Verification items for the finished model (mm, model axes). A direction names the side the tool comes from. Give positions to 0.01 mm unless a question says otherwise; leave off trailing zeros. Order: outer loops, then holes, each group sorted by start corner. A loop starts at its lowest first (then second) coordinate and runs counter-clockwise, first axis right, second up.
from build123d import *

# Parameters (mm, degrees)
BOSS_EXTRUDE1_DEPTH = 70
SKETCH3_R           = 19.5
BOSS_EXTRUDE2_DEPTH = 23
CUT_EXTRUDE1_DEPTH  = 23
CUT_EXTRUDE2_DEPTH  = 12
SKETCH4_W           = 22
SKETCH4_H           = 92.60205789
CUT_EXTRUDE3_DEPTH  = 6
SKETCH5_W           = 22
SKETCH5_H           = 56
CUT_EXTRUDE4_DEPTH  = 6


with BuildPart() as part:
    # Sketch1 → Boss-Extrude1 (new body)
    with BuildSketch(Plane(origin=(0, 0, 0), x_dir=(0, 0, -1), z_dir=(1, 0, 0))):
        Polygon((0, 0), (-149.274923862, 0), (-212.764789027, 75.664274903), (-191.31554462, 93.662327975), (-206.099659643, 111.281350166), (-245.167926242, 78.499182072), (-160, -23), (0, -23), align=None)
    extrude(amount=-BOSS_EXTRUDE1_DEPTH)

    # Sketch3 → Boss-Extrude2 (add)
    with BuildSketch(Plane(origin=(0, 166.78684827, 139.950782869), x_dir=(1, 0, 0), z_dir=(0, 0.766044443, 0.64278761))):
        with Locations((-35, -86.351225922)):
            Circle(SKETCH3_R)
        with BuildLine():
            ThreePointArc((-70, -86.351225922), (-35, -51.351225922), (0, -86.351225922))
            Line((0, -86.351225922), (-70, -86.351225922))
        make_face()
        with BuildLine():
            Line((-44.5, -86.351225922), (-54.5, -86.351225922))
            ThreePointArc((-54.5, -86.351225922), (-35, -105.851225922), (-15.5, -86.351225922))
            Line((-15.5, -86.351225922), (-25.5, -86.351225922))
            ThreePointArc((-25.5, -86.351225922), (-35, -95.851225922), (-44.5, -86.351225922))
        make_face()
        with BuildLine():
            ThreePointArc((-15.5, -86.351225922), (-35, -66.851225922), (-54.5, -86.351225922))
            Line((-54.5, -86.351225922), (-44.5, -86.351225922))
            ThreePointArc((-44.5, -86.351225922), (-35, -76.851225922), (-25.5, -86.351225922))
            Line((-25.5, -86.351225922), (-15.5, -86.351225922))
        make_face()
    extrude(amount=-BOSS_EXTRUDE2_DEPTH)

    # Sketch3_3 → Cut-Extrude1 (cut)
    with BuildSketch(Plane(origin=(0, 166.78684827, 139.950782869), x_dir=(1, 0, 0), z_dir=(0, 0.766044443, 0.64278761))):
        with BuildLine():
            Line((-25.5, -86.351225922), (-44.5, -86.351225922))
            ThreePointArc((-44.5, -86.351225922), (-35, -95.851225922), (-25.5, -86.351225922))
        make_face()
        with BuildLine():
            ThreePointArc((-25.5, -86.351225922), (-35, -76.851225922), (-44.5, -86.351225922))
            Line((-44.5, -86.351225922), (-25.5, -86.351225922))
        make_face()
    extrude(amount=-CUT_EXTRUDE1_DEPTH, mode=Mode.SUBTRACT)

    # Sketch3_4 → Cut-Extrude2 (cut)
    with BuildSketch(Plane(origin=(0, 166.78684827, 139.950782869), x_dir=(1, 0, 0), z_dir=(0, 0.766044443, 0.64278761))):
        with BuildLine():
            Line((-44.5, -86.351225922), (-54.5, -86.351225922))
            ThreePointArc((-54.5, -86.351225922), (-35, -105.851225922), (-15.5, -86.351225922))
            Line((-15.5, -86.351225922), (-25.5, -86.351225922))
            ThreePointArc((-25.5, -86.351225922), (-35, -95.851225922), (-44.5, -86.351225922))
        make_face()
        with BuildLine():
            ThreePointArc((-15.5, -86.351225922), (-35, -66.851225922), (-54.5, -86.351225922))
            Line((-54.5, -86.351225922), (-44.5, -86.351225922))
            ThreePointArc((-44.5, -86.351225922), (-35, -76.851225922), (-25.5, -86.351225922))
            Line((-25.5, -86.351225922), (-15.5, -86.351225922))
        make_face()
    extrude(amount=-CUT_EXTRUDE2_DEPTH, mode=Mode.SUBTRACT)

    # Sketch4 → Cut-Extrude3 (cut)
    with BuildSketch(Plane(origin=(0, 166.78684827, 139.950782869), x_dir=(1, 0, 0), z_dir=(0, 0.766044443, 0.64278761))):
        with Locations((-35, -91.050196977)):
            Rectangle(SKETCH4_W, SKETCH4_H)
    extrude(amount=-CUT_EXTRUDE3_DEPTH, mode=Mode.SUBTRACT)

    # Sketch5 → Cut-Extrude4 (cut)
    with BuildSketch(Plane(origin=(0, -88.287666198, 105.217143373), x_dir=(1, 0, 0), z_dir=(0, -0.64278761, 0.766044443))):
        with Locations((-35, 183.724767497)):
            Rectangle(SKETCH5_W, SKETCH5_H)
    extrude(amount=-CUT_EXTRUDE4_DEPTH, mode=Mode.SUBTRACT)


solid = part.part
(1) Section check A-A, the plane x = -28. Enter the section's corners in (y, z).
Solved:
outline: (-23, 0) - (0, 0) - (0, 149.27) - (75.66, 212.76) - (89.53, 196.24) - (97.96, 203.31) - (90.39, 212.33) - (94.99, 216.19) - (77.76, 236.71) - (34.86, 200.72) - (31, 205.32) - (-23, 160) - close; (97.79, 186.4) - (115.71, 165.05) - (128.73, 175.97) - (118.38, 188.3) - (113.79, 184.44) - (106.22, 193.47) - close
(2) Section check C-C, the plane x = -41.5. Enter the section's corners in (y, z), then the cut area to 3 significant figures.
Solved:
outline: (-23, 0) - (0, 0) - (0, 149.27) - (75.66, 212.76) - (89.21, 196.62) - (97.64, 203.69) - (90.27, 212.47) - (94.87, 216.33) - (77.76, 236.71) - (34.86, 200.72) - (31, 205.32) - (-23, 160) - close; (98.12, 186.01) - (115.77, 164.97) - (128.79, 175.9) - (118.5, 188.16) - (113.91, 184.3) - (106.54, 193.08) - close
area: 6,690 mm2
(3) Section check D-D, the plane z = 95. Enter the section's corners in (x, y).
Solved:
outline: (-70, -23) - (0, -23) - (0, 0) - (-70, 0) - close
(4) Scan lines: line 1 (Y direction, x = -57.5, z = 27.5); line 2 (Z direction, x = -59, y = 91.5); line 3 (Z direction, x = -17, y = -5). Record each from-to range of solid material in increasing order.
Solved:
line 1: y = -23 to 0
line 2: z = 193.89 to 229.67
line 3: z = 0 to 175.1
(5) Set-up check for faces 4 (the flat face through (-35.154, 123.194, 182.569)), 5 (the flat face through (-46, 65.6, 226.8)), 6 (the flat face through (-34.51, 37.302, 180.575)), 7 (the flat face through (-43.94, 99.479, 201.497)), 8 (the flat face through (-35, 0, 74)): record each of +Z, -Z, +X, -X, +Y, -Y from which the full face is reachable in a straight line by a thin tool's end or side.
Solved:
face 4: +Z, +Y
face 5: +Z
face 6: -Z, +X, -X
face 7: none
face 8: -Z, +X, -X, +Y
(6) Release check for a two-part mould opening along X. For faces 1 (the cylindrical face through (-35.77, 125.09, 172.01)), 2 (the cylindrical face through (-37.06, 91.97, 202)), 3 (the flat face through (-35, -12, 0)) record: pulls with the +X half, pulls with the -X half, needs draft (parallel to the pull), parting line crosses it, or undercut.
Solved:
face 1: parting line crosses it
face 2: undercut
face 3: needs draft
(7) Section check B-B, the plane y = 51. Enter the section's corners in (x, z), then the cut area to 3 significant figures.
Solved:
outline: (-70, 192.07) - (0, 192.07) - (0, 222.09) - (-24, 222.09) - (-24, 214.26) - (-46, 214.26) - (-46, 222.09) - (-70, 222.09) - close
area: 1,930 mm2
(8) Go/stop test with flat-tipped pins: pin 1 (8 mm diameter, centred on x = -11, y = 112.5, fed in from +Z); pin 2 (8 mm diameter, centred on x = -28.5, z = 182.5, fed in from -Y); pin 3 (2 mm diameter, centred on x = -54, y = 85, fed in from -Z). Record where each tip stops, or that it passes through.
Solved:
pin 1: stops at z = 209.41
pin 2: stops at y = -0.95
pin 3: stops at z = 200.45
